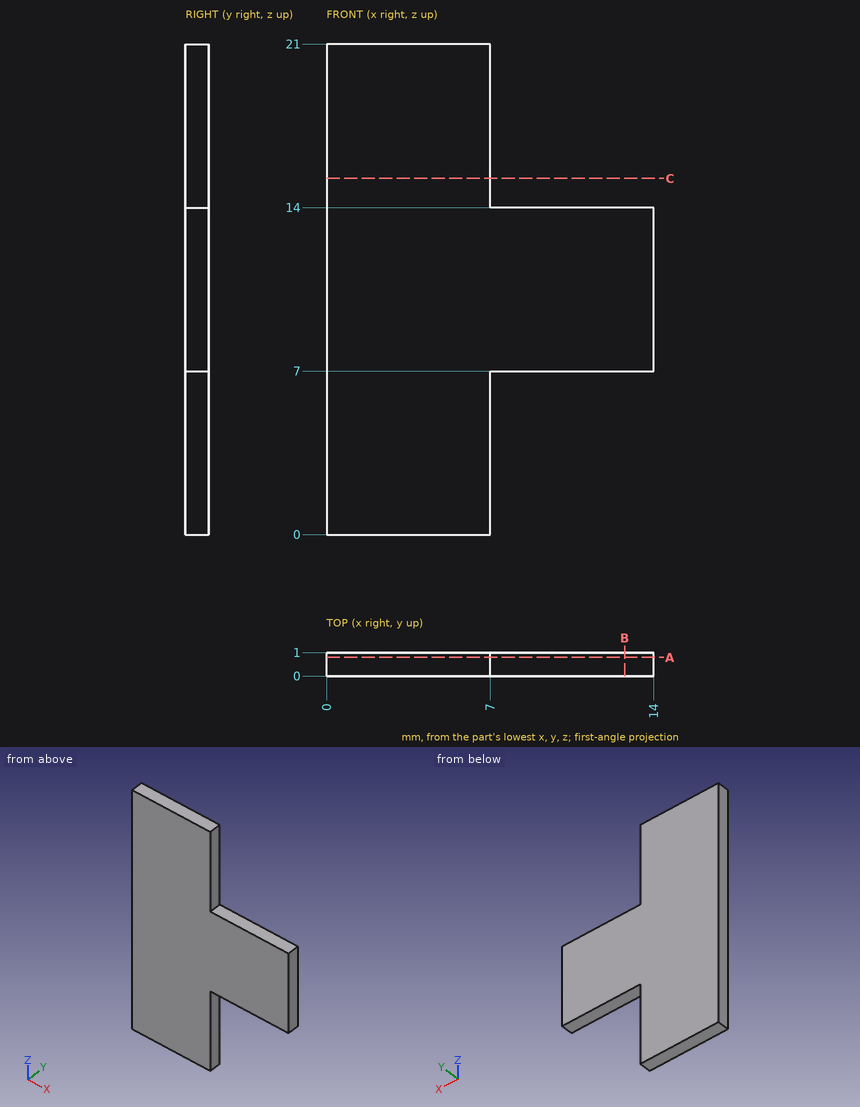
Could you check a few things on this drawing? It's one solid part, dimensions in mm from its lowest x, y, z. Round coordinates to 2 decimals unless told otherwise and drop trailing zeros. Order: outer loops, then holes, each group sorted by start corner. A loop starts at its lowest first (then second) coordinate and runs counter-clockwise, first axis right, second up. Notation, with made-up numbers: M -40,-28.5 L -3,-28.5 A12 cw -3,-14.5 Z; hole C 39.5,82.5 d7. An arc over 180 degrees is marked long. Return JSON: item names as keys, results as strings. Group by question number.
1. If we section it at A-A on y = 0.8: List the corners of the cut face in (x, z) for me, then the cut area to 3 significant figures.
2. If we section it at B-B on x = 12.75: List the corners of the cut face in (y, z) for me.
3. Please list where these lines run through material, in increasing order: probe 1 along X at (y, z) = (0.2, 3.5); probe 2 along Z at (x, y) = (7.5, 0.3).
4. If we section it at C-C on z = 15.25: List the corners of the cut face in (x, y) for me, then the cut area to 3 significant figures.
Reply:
{
 "1": {"outline": "M 0,0 L 7,0 L 7,7 L 14,7 L 14,14 L 7,14 L 7,21 L 0,21 Z", "area": "196 mm^2"},
 "2": {"outline": "M 0,7 L 1,7 L 1,14 L 0,14 Z"},
 "3": {"probe 1": "0 to 7", "probe 2": "7 to 14"},
 "4": {"outline": "M 0,0 L 7,0 L 7,1 L 0,1 Z", "area": "7.00 mm^2"}
}
